from build123d import *

# Parameters (mm, degrees)
SKETCH1_W           = 99
SKETCH1_H           = 62.5
BOSS_EXTRUDE1_DEPTH = 53.7
SKETCH2_W           = 79
SKETCH2_H           = 62.5
CUT_EXTRUDE1_DEPTH  = 50.7
SKETCH3_W           = 25
SKETCH3_H           = 62.5
BOSS_EXTRUDE2_DEPTH = 10
BOSS_EXTRUDE4_DEPTH = 3
SKETCH5_W           = 24
SKETCH5_H           = 62.5
CUT_EXTRUDE3_DEPTH  = 72
CUT_EXTRUDE4_REACH  = 96.863
SKETCH6_R           = 1
SKETCH7_R           = 2.5
CUT_EXTRUDE5_DEPTH  = 72
CUT_EXTRUDE7_DEPTH  = 50


with BuildPart() as part:
    # Sketch1 → Boss-Extrude1 (new body)
    with BuildSketch(Plane(origin=(0, 0, 0), x_dir=(1, 0, 0), z_dir=(0, 1, 0))):
        with Locations((49.5, 31.25)):
            Rectangle(SKETCH1_W, SKETCH1_H)
    extrude(amount=BOSS_EXTRUDE1_DEPTH)

    # Sketch2 → Cut-Extrude1 (cut)
    with BuildSketch(Plane(origin=(0, 53.7, 0), x_dir=(1, 0, 0), z_dir=(0, 1, 0))):
        with Locations((49.5, 31.25)):
            Rectangle(SKETCH2_W, SKETCH2_H)
    extrude(amount=-CUT_EXTRUDE1_DEPTH, mode=Mode.SUBTRACT)

    # Sketch3 → Boss-Extrude2 (add)
    with BuildSketch(Plane(origin=(0, 3, 0), x_dir=(1, 0, 0), z_dir=(0, 1, 0))):
        with Locations((64.5, 31.25)):
            Rectangle(SKETCH3_W, SKETCH3_H)
    extrude(amount=BOSS_EXTRUDE2_DEPTH)

    # Sketch4 → Boss-Extrude4 (add)
    with BuildSketch(Plane.ZY.offset(-52)):
        Polygon((-62.5, 13), (-62.5, 39), (-52.5, 39), (-52.5, 18), (-10, 18), (-10, 39), (0, 39), (0, 13), align=None)
    extrude(amount=-BOSS_EXTRUDE4_DEPTH)

    # Sketch5 → Cut-Extrude3 (cut)
    with BuildSketch(Plane.XZ):
        with Locations((12, -31.25)):
            Rectangle(SKETCH5_W, SKETCH5_H)
    extrude(amount=-CUT_EXTRUDE3_DEPTH, mode=Mode.SUBTRACT)

    # Sketch6 → Cut-Extrude4 (cut, up to next)
    with BuildSketch(Plane.ZY.offset(-52), mode=Mode.PRIVATE) as cut_extrude4_sk1:
        with Locations((-56.25, 32)):
            Circle(SKETCH6_R)
    cut_extrude4_tool1 = extrude(cut_extrude4_sk1.sketch, amount=-CUT_EXTRUDE4_REACH, mode=Mode.PRIVATE) & part.part
    # Sketch6 → Cut-Extrude4 (cut, up to next)
    with BuildSketch(Plane.ZY.offset(-52), mode=Mode.PRIVATE) as cut_extrude4_sk2:
        with Locations((-56.25, 22)):
            Circle(SKETCH6_R)
    cut_extrude4_tool2 = extrude(cut_extrude4_sk2.sketch, amount=-CUT_EXTRUDE4_REACH, mode=Mode.PRIVATE) & part.part
    # Sketch6 → Cut-Extrude4 (cut, up to next)
    with BuildSketch(Plane.ZY.offset(-52), mode=Mode.PRIVATE) as cut_extrude4_sk3:
        with Locations((-6.25, 22)):
            Circle(SKETCH6_R)
    cut_extrude4_tool3 = extrude(cut_extrude4_sk3.sketch, amount=-CUT_EXTRUDE4_REACH, mode=Mode.PRIVATE) & part.part
    # Sketch6 → Cut-Extrude4 (cut, up to next)
    with BuildSketch(Plane.ZY.offset(-52), mode=Mode.PRIVATE) as cut_extrude4_sk4:
        with Locations((-6.25, 32)):
            Circle(SKETCH6_R)
    cut_extrude4_tool4 = extrude(cut_extrude4_sk4.sketch, amount=-CUT_EXTRUDE4_REACH, mode=Mode.PRIVATE) & part.part
    add(cut_extrude4_tool1.solids().sort_by_distance((52, 32, -56.25))[0], mode=Mode.SUBTRACT)
    add(cut_extrude4_tool2.solids().sort_by_distance((52, 22, -56.25))[0], mode=Mode.SUBTRACT)
    add(cut_extrude4_tool3.solids().sort_by_distance((52, 22, -6.25))[0], mode=Mode.SUBTRACT)
    add(cut_extrude4_tool4.solids().sort_by_distance((52, 32, -6.25))[0], mode=Mode.SUBTRACT)

    # Sketch7 → Cut-Extrude5 (cut)
    with BuildSketch(Plane(origin=(99, 0, 0), x_dir=(0, 0, -1), z_dir=(1, 0, 0))):
        with Locations((40.5, 28)):
            Circle(SKETCH7_R)
    extrude(amount=-CUT_EXTRUDE5_DEPTH, mode=Mode.SUBTRACT)

    # Sketch10 → Cut-Extrude7 (cut)
    with BuildSketch(Plane(origin=(99, 0, 0), x_dir=(0, 0, -1), z_dir=(1, 0, 0))):
        with BuildLine():
            Line((0, 53.7), (0, 47.481187229))
            ThreePointArc((0, 47.481187229), (2.036166959, 51.663833041), (6.218812771, 53.7))
            Line((6.218812771, 53.7), (0, 53.7))
        make_face()
        with BuildLine():
            ThreePointArc((62.5, 46.622902441), (60.478284246, 51.575372551), (55.569083395, 53.7))
            Line((55.569083395, 53.7), (62.5, 53.7))
            Line((62.5, 53.7), (62.5, 46.622902441))
        make_face()
    extrude(amount=-CUT_EXTRUDE7_DEPTH, mode=Mode.SUBTRACT)


solid = part.part
Input: part model. Units: mm. Frame: model coordinates. A direction names the side the tool comes from. Coordinates: 2 decimals unless noted, no trailing zeros. Order: outer loops, then holes, each group sorted by start corner. A loop starts at its lowest first (then second) coordinate and runs counter-clockwise, first axis right, second up.
1. Cut plane C-C, the plane z = -12. Return loops of the section in (x, y).
Checked values:
outline: (24, 0) - (99, 0) - (99, 53.7) - (89, 53.7) - (89, 3) - (77, 3) - (77, 13) - (55, 13) - (55, 18) - (52, 18) - (52, 3) - (24, 3) - close
2. Ray query, line 1 along X through (y, z) = (33.5, -7); line 2 along Y through (x, z) = (94.25, -40.5); line 3 along Y through (x, z) = (53, -6). Return the intervals inside material, ascending.
Checked values:
line 1: x = 52 to 55, 89 to 99
line 2: y = 0 to 25.5, 30.5 to 53.7
line 3: y = 0 to 21.03, 22.97 to 31.03, 32.97 to 39
3. Cut plane D-D, the plane x = 38. Return loops of the section in (y, z).
Checked values:
outline: (0, -62.5) - (3, -62.5) - (3, 0) - (0, 0) - close
4. Access query for faces 1 (the cylindrical face through (53.48, 32.99, -6.38)), 2 (the flat face through (53, 39, -58)), 3 (the flat face through (53, 28, -10)), 4 (the cylindrical face through (94.07, 51.52, -60.53)), 5 (the flat face through (55, 17.5, -23.9)). Directions: +Z, -Z, +X, -X, +Y, -Y. A direction counts if a zero-diameter tool reaches every point of the face in a straight line with its end or side. Return the directions, or none.
Checked values:
face 1: -X
face 2: +Z, -Z, -X, +Y
face 3: -X, +Y
face 4: -Z, +X, -X, +Y
face 5: +Z, -Z, +Y
5. Contact query for flat-ended pins moving along their axis: P1, Ø4, axis at y = 29, z = -14.5, coming from the -X side; P2, Ø1.5, axis at x = 53, y = 32, coming from the +Z side; P3, Ø17.5, axis at x = 67.5, z = -39.5, coming from the +Y side; P4, Ø10, axis at y = 43.5, z = -55.5, coming from the -X side. Output: stop coordinate, or through.
Checked values:
P1: stops at x = 89
P2: stops at z = 0
P3: stops at y = 13
P4: stops at x = 52
6. Draft query along Z for faces 6 (the cylindrical face through (94.07, 51.62, -1.99)), 7 (the flat face through (53, 29, -52.5)), 8 (the cylindrical face through (53.48, 21.39, -57.04)), 9 (the flat face through (89, 29, -31)). Return one class per face: +Z half, -Z half, draft (parallel to the pull), parting line (faces both ways), or undercut.
Checked values:
face 6: +Z half
face 7: undercut
face 8: undercut
face 9: draft
7. Cut plane B-B, the plane y = 28. Return loops of the section in (x, z).
Checked values:
outline: (52, -62.5) - (55, -62.5) - (55, -52.5) - (52, -52.5) - close; (52, -10) - (55, -10) - (55, 0) - (52, 0) - close; (89, -62.5) - (99, -62.5) - (99, -43) - (89, -43) - close; (89, -38) - (99, -38) - (99, 0) - (89, 0) - close
8. Cut plane A-A, the plane y = 22. Return loops of the section in (x, z).
Checked values:
outline: (52, -62.5) - (55, -62.5) - (55, -57.25) - (52, -57.25) - close; (52, -55.25) - (55, -55.25) - (55, -52.5) - (52, -52.5) - close; (52, -10) - (55, -10) - (55, -7.25) - (52, -7.25) - close; (52, -5.25) - (55, -5.25) - (55, 0) - (52, 0) - close; (89, -62.5) - (99, -62.5) - (99, 0) - (89, 0) - close
